Design review of the part built by this model. Coordinates are the model's own, in mm. A direction names the side the tool comes from. Coordinates: 2 decimals unless noted, no trailing zeros. Loops run counter-clockwise (first coordinate to the right, second up) from the corner with the lowest first, then second, coordinate; pieces in that order, holes last. Notation, with made-up numbers: (-27, -13) -> (-4, -13) arc R32 cw to (-4, 24) -> close; hole circle Ø11 at (41, 25.5). An arc over 180 degrees is marked (long way). Answer as a JSON object with one key per item and string values.
```python
from build123d import *

# Parameters (mm, degrees)
BOSS_EXTRUDE1_DEPTH = 2
CUT_EXTRUDE1_DEPTH  = 1
BOSS_EXTRUDE2_START = 2
BOSS_EXTRUDE2_DEPTH = 10


with BuildPart() as part:
    # Sketch1 → Boss-Extrude1 (new body)
    with BuildSketch(Plane(origin=(0, 0, 0), x_dir=(1, 0, 0), z_dir=(0, 1, 0))):
        with BuildLine():
            ThreePointArc((-1.414531725, 0.4), (0, 1.47), (1.414531725, 0.4))
            Line((1.414531725, 0.4), (2.720753572, 0.4))
            ThreePointArc((2.720753572, 0.4), (0, 2.75), (-2.720753572, 0.4))
            Line((-2.720753572, 0.4), (-1.414531725, 0.4))
        make_face()
        with BuildLine():
            Line((-1.414531725, 0.4), (0, 0.4))
            Line((0, 0.4), (1.414531725, 0.4))
            ThreePointArc((1.414531725, 0.4), (0, 1.47), (-1.414531725, 0.4))
        make_face()
        with BuildLine():
            Line((1.414531725, 0.4), (0, 0.4))
            Line((0, 0.4), (-1.414531725, 0.4))
            ThreePointArc((-1.414531725, 0.4), (-1.47, 0), (-1.414531725, -0.4))
            Line((-1.414531725, -0.4), (1.414531725, -0.4))
            ThreePointArc((1.414531725, -0.4), (1.4560669, -0.201913799), (1.47, 0))
            ThreePointArc((1.47, 0), (1.4560669, 0.201913799), (1.414531725, 0.4))
        make_face()
        with BuildLine():
            Line((1.414531725, -0.4), (-1.414531725, -0.4))
            ThreePointArc((-1.414531725, -0.4), (0, -1.47), (1.414531725, -0.4))
        make_face()
        with BuildLine():
            ThreePointArc((1.414531725, -0.4), (0, -1.47), (-1.414531725, -0.4))
            Line((-1.414531725, -0.4), (-2.720753572, -0.4))
            ThreePointArc((-2.720753572, -0.4), (0, -2.75), (2.720753572, -0.4))
            Line((2.720753572, -0.4), (1.414531725, -0.4))
        make_face()
        with BuildLine():
            Line((2.720753572, 0.4), (1.414531725, 0.4))
            ThreePointArc((1.414531725, 0.4), (1.4560669, 0.201913799), (1.47, 0))
            ThreePointArc((1.47, 0), (1.4560669, -0.201913799), (1.414531725, -0.4))
            Line((1.414531725, -0.4), (2.720753572, -0.4))
            ThreePointArc((2.720753572, -0.4), (2.742678647, -0.200533883), (2.75, 0))
            ThreePointArc((2.75, 0), (2.742678647, 0.200533883), (2.720753572, 0.4))
        make_face()
        with BuildLine():
            ThreePointArc((-1.414531725, -0.4), (-1.47, 0), (-1.414531725, 0.4))
            Line((-1.414531725, 0.4), (-2.720753572, 0.4))
            ThreePointArc((-2.720753572, 0.4), (-2.75, 0), (-2.720753572, -0.4))
            Line((-2.720753572, -0.4), (-1.414531725, -0.4))
        make_face()
    extrude(amount=BOSS_EXTRUDE1_DEPTH)

    # Sketch1<3> → Cut-Extrude1 (cut)
    with BuildSketch(Plane(origin=(0, 0, 0), x_dir=(1, 0, 0), z_dir=(0, 1, 0))):
        with BuildLine():
            Line((2.720753572, 0.4), (1.414531725, 0.4))
            ThreePointArc((1.414531725, 0.4), (1.4560669, 0.201913799), (1.47, 0))
            ThreePointArc((1.47, 0), (1.4560669, -0.201913799), (1.414531725, -0.4))
            Line((1.414531725, -0.4), (2.720753572, -0.4))
            ThreePointArc((2.720753572, -0.4), (2.742678647, -0.200533883), (2.75, 0))
            ThreePointArc((2.75, 0), (2.742678647, 0.200533883), (2.720753572, 0.4))
        make_face()
        with BuildLine():
            ThreePointArc((-1.414531725, -0.4), (-1.47, 0), (-1.414531725, 0.4))
            Line((-1.414531725, 0.4), (-2.720753572, 0.4))
            ThreePointArc((-2.720753572, 0.4), (-2.75, 0), (-2.720753572, -0.4))
            Line((-2.720753572, -0.4), (-1.414531725, -0.4))
        make_face()
        with BuildLine():
            Line((1.414531725, 0.4), (0, 0.4))
            Line((0, 0.4), (-1.414531725, 0.4))
            ThreePointArc((-1.414531725, 0.4), (-1.47, 0), (-1.414531725, -0.4))
            Line((-1.414531725, -0.4), (1.414531725, -0.4))
            ThreePointArc((1.414531725, -0.4), (1.4560669, -0.201913799), (1.47, 0))
            ThreePointArc((1.47, 0), (1.4560669, 0.201913799), (1.414531725, 0.4))
        make_face()
    extrude(amount=CUT_EXTRUDE1_DEPTH, mode=Mode.SUBTRACT)

    # Sketch1<4> → Boss-Extrude2 (add)
    with BuildSketch(Plane(origin=(0, 0, 0), x_dir=(1, 0, 0), z_dir=(0, 1, 0)).offset(BOSS_EXTRUDE2_START)):
        with BuildLine():
            Line((-1.414531725, 0.4), (0, 0.4))
            Line((0, 0.4), (1.414531725, 0.4))
            ThreePointArc((1.414531725, 0.4), (0, 1.47), (-1.414531725, 0.4))
        make_face()
        with BuildLine():
            Line((1.414531725, 0.4), (0, 0.4))
            Line((0, 0.4), (-1.414531725, 0.4))
            ThreePointArc((-1.414531725, 0.4), (-1.47, 0), (-1.414531725, -0.4))
            Line((-1.414531725, -0.4), (1.414531725, -0.4))
            ThreePointArc((1.414531725, -0.4), (1.4560669, -0.201913799), (1.47, 0))
            ThreePointArc((1.47, 0), (1.4560669, 0.201913799), (1.414531725, 0.4))
        make_face()
        with BuildLine():
            Line((1.414531725, -0.4), (-1.414531725, -0.4))
            ThreePointArc((-1.414531725, -0.4), (0, -1.47), (1.414531725, -0.4))
        make_face()
    extrude(amount=BOSS_EXTRUDE2_DEPTH)


solid = part.part
```
1) Add section D-D, the plane x = -1.15. Give the boundary of the cut face in (y, z).
Completed:
{"outline": "(0, -2.5) -> (2, -2.5) -> (2, -0.92) -> (12, -0.92) -> (12, 0.92) -> (2, 0.92) -> (2, 2.5) -> (0, 2.5) -> (0, 0.4) -> (1, 0.4) -> (1, -0.4) -> (0, -0.4) -> close"}
2) Wall thickness on probe 1 along Y at (x, z) = (0.55, 1.8); probe 2 along Y at (x, z) = (-1.05, -0.2); probe 3 along Z at (x, y) = (0.05, 11.5): over which ranges is each line inside the solid? List them lowest first.
Completed:
{"probe 1": "0 to 2", "probe 2": "1 to 12", "probe 3": "-1.47 to 1.47"}
3) Add section C-C, the plane z = 1.15. Give the boundary of the cut face in (x, y), and give its area (3 significant figures).
Completed:
{"outline": "(-2.5, 0) -> (2.5, 0) -> (2.5, 2) -> (0.92, 2) -> (0.92, 12) -> (-0.92, 12) -> (-0.92, 2) -> (-2.5, 2) -> close", "area": "28.3 mm²"}
4) Add section B-B, the plane y = 7.5. Give the boundary of the cut face in (x, z).
Completed:
{"outline": "circle Ø2.94 at (0, 0)"}
5) Clearance check with flat-ended pins moving along their axes: pin 1 Ø3 at (y, z) = (7, -0.5) entering from -X; pin 2 Ø3 at (x, z) = (-1.5, 1) entering from -Y; pin 3 Ø2 at (x, y) = (1, 9.5) entering from +Z; pin 4 Ø0.5 at (x, y) = (1, 0.5) entering from -Z. State where each tip first meets the part, or that it passes through.
Completed:
{"pin 1": "x = -1.47", "pin 2": "y = 0", "pin 3": "z = 1.47", "pin 4": "z = -2.65"}
6) For faces 1 (the flat face through (0, 0, -1)), 2 (the flat face through (1.2, 2, 1.2)), 3 (the flat face through (0, 1, 0)), list the 3-axis set-ups (+Z, -Z, +X, -X, +Y, -Y) from which the entire face can be reached by the end or side of a thin tool; tool diameter is ignored.
Completed:
{"face 1": "+Z, -Z, +X, -X, -Y", "face 2": "+Y", "face 3": "+X, -X, -Y"}
7) Add section A-A, the plane x = -2.2. Give the boundary of the cut face in (y, z).
Completed:
{"outline": "(0, -1.65) -> (2, -1.65) -> (2, 1.65) -> (0, 1.65) -> (0, 0.4) -> (1, 0.4) -> (1, -0.4) -> (0, -0.4) -> close"}
